Autodesk Inventor part; units mm, degrees
ref_plane "YZ Plane" through (0, 0, 0) normal (1, 0, 0) x (0, 1, 0)
ref_plane "XZ Plane" through (0, 0, 0) normal (0, 1, 0) x (-1, 0, 0)
ref_plane "XY Plane" through (0, 0, 0) normal (0, 0, 1) x (1, 0, 0)
sketch "スケッチ1" plane through (0, 0, 0) normal (0, 0, 1) x (1, 0, 0)
  circle A0 centre (0, 0) radius 1.5
  dimension "d0" = 3
extrude "押し出し1" add sketch "スケッチ1" along normal blind 20
thread "ねじ1"
sketch "スケッチ2" plane through (0, 0, 20) normal (0, 0, 1) x (1, 0, 0)
  circle A0 centre (0, 0) radius 3
  dimension "d5" = 6
extrude "押し出し2" add sketch "スケッチ2" against normal blind 1.75
chamfer "面取り1" distance 1.5 angle 45 1 edges at (-3, 0, 18.25)
sketch "スケッチ3" plane through (0, 0, 20) normal (0, 0, 1) x (1, 0, 0)
  line L0 (0, 1.1547) -> (1, 0.5774)
  line L1 (1, 0.5774) -> (1, -0.5774)
  line L2 (1, -0.5774) -> (0, -1.1547)
  line L3 (0, -1.1547) -> (-1, -0.5774)
  line L4 (-1, -0.5774) -> (-1, 0.5774)
  line L5 (-1, 0.5774) -> (0, 1.1547)
  point P0 (0, 0)
  point P1 (0, 0)
  dimension "d11" = 2
extrude "押し出し3" cut sketch "スケッチ3" against normal blind 1.5
properties part number "m3皿ネジ　２０" material "鉄 灰色"
Check sheet for the modelled part. Datum: model origin and axes. Units: mm. A direction names the side the tool comes from. Round coordinates to 2 decimals unless told otherwise and drop trailing zeros. Loops run counter-clockwise (first coordinate to the right, second up) from the corner with the lowest first, then second, coordinate; pieces in that order, holes last. Notation, with made-up numbers: (-7.5, -25) -> (20.5, -25) arc R20 ccw to (20.5, -10) -> close; hole circle Ø11 at (36, 16). An arc over 180 degrees is marked (long way). Put each result on its own line as item: value. Start each with the question number.
1. Access from +Z, -Z, +X, -X, +Y, -Y to the whole of each face (thin tool, end or side, straight path). Record for faces 1 (the face through (1.3, 0, 20)), 2 (the face through (-0.49, -0.87, 19.26)).
2. Scan lines: probe 1 along Z at (x, y) = (0.1, 0.55); probe 2 along X at (y, z) = (-0.5, 8.5); probe 3 along Y at (x, z) = (-0.9, 16.75). Record each from-to range of solid material in increasing order.
3. Gauge pin test, flat ends, axial feed: pin 1 (3 mm diameter, centred on x = -0.5, z = 16, fed in from +Y); pin 2 (1.5 mm diameter, centred on y = 1.5, z = 5.5, fed in from -X). Record the tip position at first contact, or that the pin passes through.
4. Draft check along X on faces 3 (the face through (-1, 0, 19)), 4 (the face through (0, 0, 0)), 5 (the face through (-1.5, -0.07, 9)). Enter one of: +X half, -X half, draft (parallel to the pull), parting line (faces both ways), or undercut.
5. Section check B-B (z = 16). Enter the section's corners in (x, y).
Findings:
1. face 1: +Z, +X, -X, +Y, -Y
1. face 2: +Z
2. probe 1: z = 0 to 18.5
2. probe 2: x = -1.41 to 1.41
2. probe 3: y = -1.2 to 1.2
3. pin 1: stops at y = 1.5
3. pin 2: stops at x = -1.3
4. face 3: undercut
4. face 4: draft
4. face 5: parting line
5. outline: circle Ø3 at (0, 0)
